Source: CAD feature listing. Evaluate the final solid. Frame: model axes, mm. A direction names the side the tool comes from. Give positions to 0.01 mm unless a question says otherwise; leave off trailing zeros. Loops run counter-clockwise (first coordinate to the right, second up) from the corner with the lowest first, then second, coordinate; pieces in that order, holes last. Notation, with made-up numbers: M 41,20 L 95,20 A21 ccw 95,32 Z; hole C 84,-37 d1. An arc over 180 degrees is marked long. Put each result on its own line as item: value. Start each with the question number.
```python
from build123d import *

# Parameters (mm, degrees)
F0_R          = 18.9135358378
F0_R_2        = 11.1250506431
F1_DEPTH      = 4
F1_DEPTH_BACK = 4
F2_R          = 3.8258628395
F3_DEPTH      = 28
F3_DEPTH_BACK = 28
F4_R          = 3.8258764398
F5_DEPTH      = 11.5
F5_DEPTH_BACK = 11.5
F6_R          = 3.830099353
F7_DEPTH      = 25
F7_DEPTH_BACK = 25
F8_R          = 3.9189417201
F9_DEPTH      = 11.5
F9_DEPTH_BACK = 11.5


with BuildPart() as f1:
    # F0 (on Front) → F1 (new body, two sides)
    with BuildSketch(Plane.XZ) as f1_sk:
        Circle(F0_R)
        Circle(F0_R_2, mode=Mode.SUBTRACT)
    extrude(amount=F1_DEPTH)
    extrude(f1_sk.sketch, amount=-F1_DEPTH_BACK)

    # F2 (on Top) → F3 (join, two sides)
    with BuildSketch(Plane.XY) as f3_sk:
        Circle(F2_R)
    extrude(amount=F3_DEPTH)
    extrude(f3_sk.sketch, amount=-F3_DEPTH_BACK)

    # F4 (on Top) → F5 (cut, two sides)
    with BuildSketch(Plane.XY) as f5_sk:
        Circle(F4_R)
    extrude(amount=-F5_DEPTH, mode=Mode.SUBTRACT)
    extrude(f5_sk.sketch, amount=F5_DEPTH_BACK, mode=Mode.SUBTRACT)

    # F6 (on Right) → F7 (join, two sides)
    with BuildSketch(Plane.YZ) as f7_sk:
        Circle(F6_R)
    extrude(amount=F7_DEPTH)
    extrude(f7_sk.sketch, amount=-F7_DEPTH_BACK)

    # F8 (on Right) → F9 (cut, two sides)
    with BuildSketch(Plane.YZ) as f9_sk:
        Circle(F8_R)
    extrude(amount=-F9_DEPTH, mode=Mode.SUBTRACT)
    extrude(f9_sk.sketch, amount=F9_DEPTH_BACK, mode=Mode.SUBTRACT)


solid = f1.part
```
1. Set-up query: faces 5 (the face through (0, 0, -11.5)), 6 (the face through (21.715, -3.826, 0.168)), 7 (the face through (-0.829, -3.735, -23.195)), 8 (the face through (-0.829, -3.735, 23.195)). Return all of +Z, -Z, +X, -X, +Y, -Y with unobstructed straight access to the full face (end or side cutting, diameter ignored); none if empty.
2. Pull-direction query (Y, two-part tool) for faces 1 (the face through (0, 0, -28)), 2 (the face through (8, 4, -8)), 3 (the face through (-21.715, -3.826, 0.168)), 4 (the face through (11.19, 3.62, -1.5)); classes: released by +Y, released by -Y, zero draft, split by the parting line, or undercut.
3. Ray query, line 1 (Z direction, x = 0.5, y = -1.5); line 2 (Y direction, x = 0, z = -11.2); line 3 (X direction, y = 0, z = -11.2). Return the intervals inside material, ascending.
4. Section A-A, the plane z = 0. Output: boundary loops of the cut face in (x, y), plus the area to 3 significant figures.
5. Contact query for flat-ended pins moving along their axis: pin 1 (1.5 mm diameter, centred on x = -8.5, y = -1.5, fed in from -Z); pin 2 (18 mm diameter, centred on x = 0, z = 0, fed in from -Y); pin 3 (1 mm diameter, centred on x = -12.5, y = -1.5, fed in from -Z); pin 4 (12 mm diameter, centred on x = -3.5, z = 9.5, fed in from -Y). Output: stop coordinate, or through.
6. Section C-C, the plane x = 0. Output: boundary loops of the cut face in (y, z), plus the area to 3 significant figures.
7. Section D-D, the plane z = 6. Output: boundary loops of the cut face in (x, y), plus the area to 3 significant figures.
Results found:
1. face 5: none
1. face 6: +X
1. face 7: -Z
1. face 8: +Z
2. face 1: zero draft
2. face 2: released by +Y
2. face 3: split by the parting line
2. face 4: undercut
3. line 1: -28 to -11.5, 11.5 to 28
3. line 2: -4 to -3.83, 3.83 to 4
3. line 3: -15.24 to -3.83, 3.83 to 15.24
4. outline: M -25,-3.83 L -18.91,-3.83 L -18.91,-4 L -11.13,-4 L -11.13,-3.92 L -11.5,-3.92 L -11.5,3.92 L -11.13,3.92 L -11.13,4 L -18.91,4 L -18.91,3.83 L -25,3.83 Z; M 11.13,-4 L 18.91,-4 L 18.91,-3.83 L 25,-3.83 L 25,3.83 L 18.91,3.83 L 18.91,4 L 11.13,4 L 11.13,3.92 L 11.5,3.92 L 11.5,-3.92 L 11.13,-3.92 Z
4. area: 212 mm²
5. pin 1: z = -17.25
5. pin 2: through
5. pin 3: z = -14.62
5. pin 4: y = -4
6. outline: M -4,-18.91 L -3.83,-18.91 L -3.83,-28 L 3.83,-28 L 3.83,-18.91 L 4,-18.91 L 4,-11.13 L 3.83,-11.13 L 3.83,-11.5 L -3.83,-11.5 L -3.83,-11.13 L -4,-11.13 Z; M -4,11.13 L -3.83,11.13 L -3.83,11.5 L 3.83,11.5 L 3.83,11.13 L 4,11.13 L 4,18.91 L 3.83,18.91 L 3.83,28 L -3.83,28 L -3.83,18.91 L -4,18.91 Z
6. area: 258 mm²
7. outline: M -17.94,-4 L -9.37,-4 L -9.37,4 L -17.94,4 Z; M 9.37,-4 L 17.94,-4 L 17.94,4 L 9.37,4 Z
7. area: 137 mm²
